CAD build for the part. Positions are in the model's coordinates, mm. A direction names the side the tool comes from. Give positions to 0.01 mm unless a question says otherwise; leave off trailing zeros. Loops run counter-clockwise (first coordinate to the right, second up) from the corner with the lowest first, then second, coordinate; pieces in that order, holes last.
Item 1: Probe probe 1 along Z at (x, y) = (1.3, 5.5); probe 2 along Z at (x, y) = (2.5, 18); probe 3 along Z at (x, y) = (0.5, -1). List the from-to ranges inside material, lowest first.
Item 2: Saw through at D-D on x = 2.45. Give the cut face in (y, z) (1 decimal).
Item 3: Mould opens along Z. For faces 1 (the flat face through (2, 3.683, -4)), 2 (the flat face through (2, 8, -16.764)), 3 (the cylindrical face through (1.565, 34.185, -1.189)), 4 (the flat face through (2, 0, 5)) say: released by +Z, released by -Z, zero draft, split by the parting line, or undercut.
Item 4: Saw through at A-A on y = 2. Give the cut face in (x, z) (3 decimals).
Item 5: Which spindle directions (+Z, -Z, +X, -X, +Y, -Y) get a long thin tool onto all of the face, cutting with end or side? Do faces 5 (the flat face through (2, -2, 10.541)), 6 (the flat face through (2, 6.477, -2)), 7 (the flat face through (2, -3.175, 12)). Say none if no direction does.
Item 6: Drop flat-ended pins along their axis: P1, Ø0.8, axis at x = 1.5, z = -3.5, coming from the +Y side; P2, Ø1.5, axis at x = 3, y = 20, coming from the -Z side; P3, Ø4, axis at y = 21, z = 0, coming from the +X side. Give the stop position or say it passes through.
Item 7: Saw through at C-C on y = 23. Give the cut face in (x, z) (3 decimals).
Item 8: Saw through at B-B on z = 1. Give the cut face in (x, y) (3 decimals), plus the area to 3 significant figures.
from build123d import *

# Parameters (mm, degrees)
SKETCH1_R           = 6
SKETCH1_R_2         = 1.5875
BOSS_EXTRUDE1_DEPTH = 3.175


with BuildPart() as part:
    # Sketch1 → Boss-Extrude1 (new body)
    with BuildSketch(Plane(origin=(0, 0, 0), x_dir=(0, 0, -1), z_dir=(1, 0, 0))):
        with BuildLine():
            Line((-13.716, -3.175), (-13.716, 18.94882794))
            ThreePointArc((-13.716, 18.94882794), (1.524, 34.18882794), (16.764, 18.94882794))
            Line((16.764, 18.94882794), (16.764, -3.175))
            Line((16.764, -3.175), (13.589, -3.175))
            Line((13.589, -3.175), (13.589, 0))
            Line((13.589, 0), (3.048, 0))
            Line((3.048, 0), (3.048, 3.683))
            Line((3.048, 3.683), (4.699, 3.683))
            Line((4.699, 3.683), (4.699, 6.477))
            Line((4.699, 6.477), (-1.651, 6.477))
            Line((-1.651, 6.477), (-1.651, 3.683))
            Line((-1.651, 3.683), (0, 3.683))
            Line((0, 3.683), (0, 0))
            Line((0, 0), (-10.541, 0))
            Line((-10.541, 0), (-10.541, -3.175))
            Line((-10.541, -3.175), (-13.716, -3.175))
        make_face()
        with Locations((1.524, 19.423957259)):
            Circle(SKETCH1_R, mode=Mode.SUBTRACT)
        with Locations((-7.476, 19.423957259)):
            Circle(SKETCH1_R_2, mode=Mode.SUBTRACT)
        with Locations((10.524, 19.423957259)):
            Circle(SKETCH1_R_2, mode=Mode.SUBTRACT)
    extrude(amount=BOSS_EXTRUDE1_DEPTH)


solid = part.part
Results below:
1. probe 1: z = -16.76 to -4.7, 1.65 to 13.72
1. probe 2: z = -16.76 to -11.23, -9.82 to -7.35, 4.3 to 6.77, 8.18 to 13.72
1. probe 3: z = -16.76 to -13.59, 10.54 to 13.72
2. outline: (-3.2, -16.8) - (18.9, -16.8) arc R15.2 ccw to (18.9, 13.7) - (-3.2, 13.7) - (-3.2, 10.5) - (0, 10.5) - (0, 0) - (3.7, 0) - (3.7, 1.7) - (6.5, 1.7) - (6.5, -4.7) - (3.7, -4.7) - (3.7, -3) - (0, -3) - (0, -13.6) - (-3.2, -13.6) - close; hole circle Ø12 at (19.4, -1.5); hole circle Ø3.2 at (19.4, -10.5); hole circle Ø3.2 at (19.4, 7.5)
3. face 1: undercut
3. face 2: released by -Z
3. face 3: split by the parting line
3. face 4: undercut
4. outline: (0, -16.764) - (3.175, -16.764) - (3.175, -3.048) - (0, -3.048) - close; (0, 0) - (3.175, 0) - (3.175, 13.716) - (0, 13.716) - close
5. face 5: +X, -X, -Y
5. face 6: +X, -X
5. face 7: +Z, -Z, +X, -X, -Y
6. P1: stops at y = 34.11
6. P2: stops at z = -16.76
6. P3: passes through
7. outline: (0, -16.216) - (3.175, -16.216) - (3.175, -6.342) - (0, -6.342) - close; (0, 3.294) - (3.175, 3.294) - (3.175, 13.168) - (0, 13.168) - close
8. outline: (0, 0) - (3.175, 0) - (3.175, 3.683) - (0, 3.683) - close; (0, 6.477) - (3.175, 6.477) - (3.175, 13.981) - (0, 13.981) - close; (0, 24.867) - (3.175, 24.867) - (3.175, 33.978) - (0, 33.978) - close
8. area: 64.4 mm2
